Check sheet for the drawn part. Datum: minimum x, y, z corner. Units: mm. Coordinates: 2 decimals unless noted, no trailing zeros. Order: outer loops, then holes, each group sorted by start corner. A loop starts at its lowest first (then second) coordinate and runs counter-clockwise, first axis right, second up. Notation, with made-up numbers: M 70,60.25 L 81,60.25 A22 cw 81,75.25 Z; hole C -32.75,60 d9. An arc over 180 degrees is marked long. Use one line per item in the form item = value. Start each with the question number.
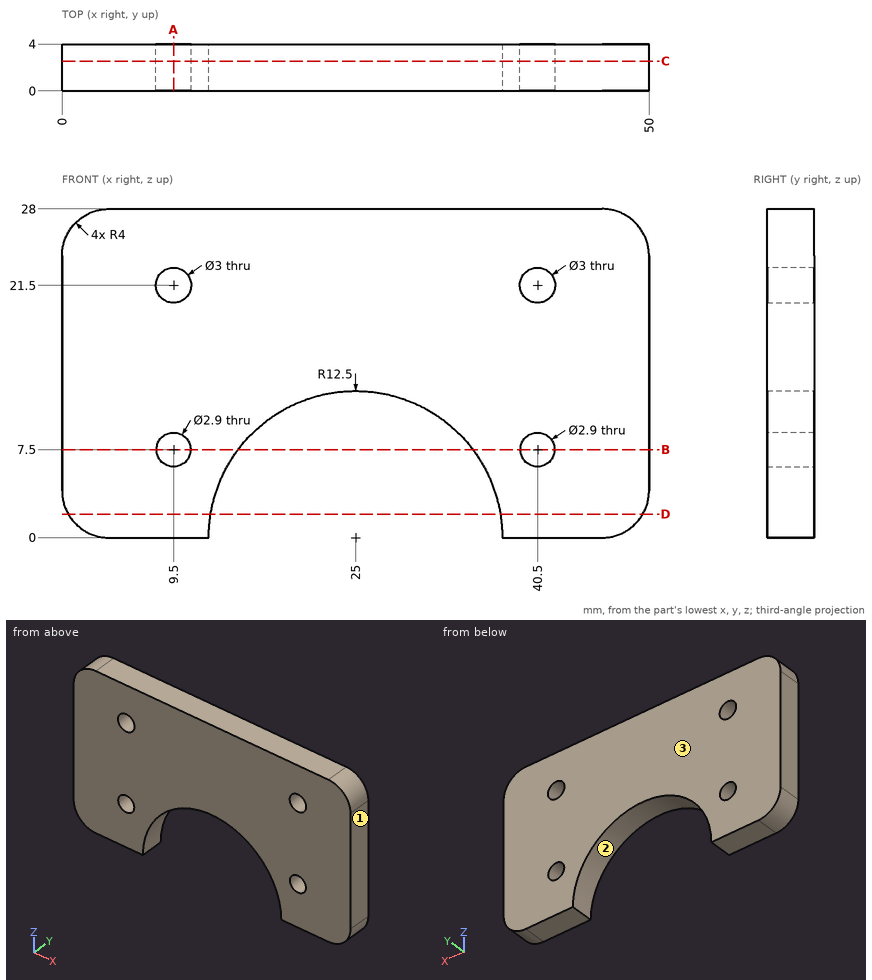
1. Cross-section at A-A on x = 9.5. Enter the section's corners in (y, z).
2. Material ranges on line 1 along X through (y, z) = (2.3, 21.5); line 2 along X through (y, z) = (1, 8.5); line 3 along X through (y, z) = (3, 7.5), recorded low to high.
3. Cross-section at B-B on z = 7.5. Enter the section's corners in (x, y), and give its area (3 significant figures).
4. Cross-section at C-C on y = 2.55. Enter the section's corners in (x, z), and give its area (3 significant figures).
5. Cross-section at D-D on z = 2. Enter the section's corners in (x, y), and give its area (3 significant figures).
6. Release check for a two-part mould opening along X. For the marked faces 1, 2 and 3 record: pulls with the +X half, pulls with the -X half, needs draft (parallel to the pull), parting line crosses it, or undercut.
Final values:
q1.outline = M 0,0 L 4,0 L 4,6.05 L 0,6.05 Z; M 0,8.95 L 4,8.95 L 4,20 L 0,20 Z; M 0,23 L 4,23 L 4,28 L 0,28 Z
q2.line_1 = 0 to 8, 11 to 39, 42 to 50
q2.line_2 = 0 to 8.45, 10.55 to 15.83, 34.17 to 39.45, 41.55 to 50
q2.line_3 = 0 to 8.05, 10.95 to 15, 35 to 39.05, 41.95 to 50
q3.outline = M 0,0 L 8.05,0 L 8.05,4 L 0,4 Z; M 10.95,0 L 15,0 L 15,4 L 10.95,4 Z; M 35,0 L 39.05,0 L 39.05,4 L 35,4 Z; M 41.95,0 L 50,0 L 50,4 L 41.95,4 Z
q3.area = 96.8 mm2
q4.outline = M 0,4 A4 ccw 4,0 L 12.5,0 A12.5 cw 37.5,0 L 46,0 A4 ccw 50,4 L 50,24 A4 ccw 46,28 L 4,28 A4 ccw 0,24 Z; hole C 9.5,21.5 d3; hole C 9.5,7.5 d2.9; hole C 40.5,21.5 d3; hole C 40.5,7.5 d2.9
q4.area = 1,110 mm2
q5.outline = M 0.54,0 L 12.66,0 L 12.66,4 L 0.54,4 Z; M 37.34,0 L 49.46,0 L 49.46,4 L 37.34,4 Z
q5.area = 97.0 mm2
q6.face_1 = pulls with the +X half
q6.face_2 = undercut
q6.face_3 = needs draft
